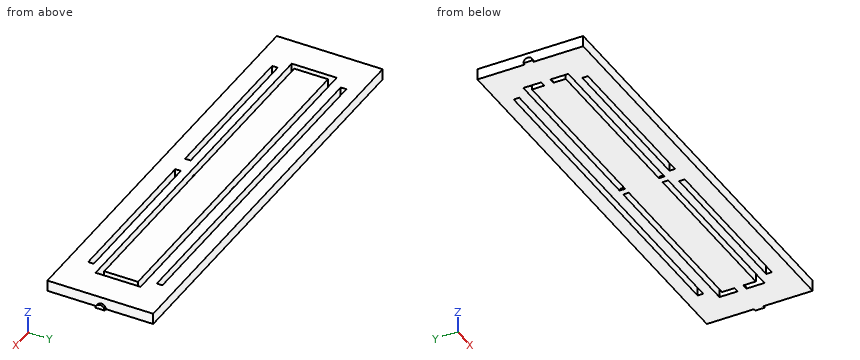
```python
from build123d import *

# Parameters (mm, degrees)
F3_DEPTH      = 24
F3_DEPTH_BACK = 23
F2_W          = 150.6
F2_H          = 2.5
F2_W_2        = 71.3
F2_W_3        = 160.6
F2_H_2        = 20
F2_W_4        = 155.6
F2_H_3        = 15
F4_DEPTH      = 4.9
F7_DEPTH      = 95
F7_DEPTH_BACK = 95
F8_DEPTH      = 12
F8_DEPTH_BACK = 12
F9_DEPTH      = 4.75


with BuildPart() as f3:
    # F1 (on Front) → F3 (new body, two sides)
    with BuildSketch(Plane.XZ) as f3_sk:
        Polygon((-93.9166666667, 0), (0, 0), (93.9166666667, 0), (93.9166666667, 4.9), (0, 4.9), (-93.9166666667, 4.9), align=None)
    extrude(amount=F3_DEPTH)
    extrude(f3_sk.sketch, amount=-F3_DEPTH_BACK)

    # F2 (on Top) → F4 (cut, through all)
    with BuildSketch(Plane.XY):
        with Locations((0, 15.75)):
            Rectangle(F2_W, F2_H)
        with Locations((39.65, -14.75)):
            Rectangle(F2_W_2, F2_H)
        with Locations((-39.65, -14.75)):
            Rectangle(F2_W_2, F2_H)
        Rectangle(F2_W_3, F2_H_2)
        Rectangle(F2_W_4, F2_H_3, mode=Mode.SUBTRACT)
    extrude(amount=F4_DEPTH, mode=Mode.SUBTRACT)

    # F6 (on Right) → F7 (join, two sides)
    with BuildSketch(Plane.YZ) as f7_sk:
        with BuildLine():
            Line((-2, 0), (2, 0))
            ThreePointArc((2, 0), (0, 2), (-2, 0))
        make_face()
    extrude(amount=F7_DEPTH)
    extrude(f7_sk.sketch, amount=-F7_DEPTH_BACK)

    # F0 (on Front) → F8 (join, two sides)
    with BuildSketch(Plane.XZ) as f8_sk:
        with BuildLine():
            Line((0, 1.5), (0, 0))
            Line((0, 0), (1.5, 0))
            ThreePointArc((1.5, 0), (1.0606601718, 1.0606601718), (0, 1.5))
        make_face()
        with BuildLine():
            ThreePointArc((0, 1.5), (-1.0606601718, 1.0606601718), (-1.5, 0))
            Line((-1.5, 0), (0, 0))
            Line((0, 0), (0, 1.5))
        make_face()
    extrude(amount=F8_DEPTH)
    extrude(f8_sk.sketch, amount=-F8_DEPTH_BACK)

    # F2 (on Top) → F9 (join)
    with BuildSketch(Plane.XY):
        Rectangle(F2_W_4, F2_H_3)
    extrude(amount=F9_DEPTH)


solid = f3.part
```
Design review of the part built by this model. Coordinates are the model's own, in mm. Give positions to 0.01 mm unless a question says otherwise; leave off trailing zeros. Loops run counter-clockwise (first coordinate to the right, second up) from the corner with the lowest first, then second, coordinate; pieces in that order, holes last. Notation, with made-up numbers: (-20, 88) -> (8, 88) arc R16 ccw to (8, 109) -> close; hole circle Ø1 at (71.25, 49). An arc over 180 degrees is marked (long way). One line per item, written item: value.
Q1. For pin 1 Ø2.5 at (y, z) = (-3, 2.5) entering from -X; pin 2 Ø5 at (x, y) = (-48, -15.5) entering from -Z; pin 3 Ø2 at (y, z) = (-14.5, 3.5) entering from +X, all flat-tipped, find the tip position at first contact; note any pin that passes through.
Numbers:
pin 1: stops at x = -93.92
pin 2: stops at z = 0
pin 3: stops at x = 93.92
Q2. We need section A-A on z = 4.1. Give the boundary of the cut face in (x, y).
Numbers:
outline: (-93.92, -24) -> (93.92, -24) -> (93.92, 23) -> (-93.92, 23) -> close; (-77.8, -7.5) -> (77.8, -7.5) -> (77.8, 7.5) -> (-77.8, 7.5) -> close; hole (-80.3, -10) -> (80.3, -10) -> (80.3, 10) -> (-80.3, 10) -> close; hole (-75.3, -16) -> (-4, -16) -> (-4, -13.5) -> (-75.3, -13.5) -> close; hole (-75.3, 14.5) -> (75.3, 14.5) -> (75.3, 17) -> (-75.3, 17) -> close; hole (4, -16) -> (75.3, -16) -> (75.3, -13.5) -> (4, -13.5) -> close
Q3. For L1, parallel to X at y = 4, z = 1.95; L2, parallel to Y at x = 31, z = 4.05; L3, parallel to Y at x = -2, z = 1.8, list the stretches that pass through material, from the lowest coordinate up.
Numbers:
L1: x = -93.92 to -80.3, -77.8 to 77.8, 80.3 to 93.92
L2: y = -24 to -16, -13.5 to -10, -7.5 to 7.5, 10 to 14.5, 17 to 23
L3: y = -24 to -10, -7.5 to 7.5, 10 to 14.5, 17 to 23
Q4. We need section C-C on y = 0. Give the boundary of the cut face in (x, z), and give its area (3 significant figures).
Numbers:
outline: (-95, 0) -> (95, 0) -> (95, 2) -> (93.92, 2) -> (93.92, 4.9) -> (80.3, 4.9) -> (80.3, 2) -> (77.8, 2) -> (77.8, 4.9) -> (-77.8, 4.9) -> (-77.8, 2) -> (-80.3, 2) -> (-80.3, 4.9) -> (-93.92, 4.9) -> (-93.92, 2) -> (-95, 2) -> close
area: 910 mm^2
Q5. We need section B-B on x = 9.5. Give the boundary of the cut face in (y, z).
Numbers:
outline: (-24, 0) -> (-16, 0) -> (-16, 4.9) -> (-24, 4.9) -> close; (-13.5, 0) -> (-10, 0) -> (-10, 4.9) -> (-13.5, 4.9) -> close; (-7.5, 0) -> (7.5, 0) -> (7.5, 4.9) -> (-7.5, 4.9) -> close; (10, 0) -> (14.5, 0) -> (14.5, 4.9) -> (10, 4.9) -> close; (17, 0) -> (23, 0) -> (23, 4.9) -> (17, 4.9) -> close
